Build history of the part. All positions in model axes, mm. A direction names the side the tool comes from. Round coordinates to 2 decimals unless told otherwise and drop trailing zeros. Write each loop counter-clockwise with the first axis right and the second up, starting at its lowest first coordinate (ties: lowest second). Pieces come first, ordered by that corner, then holes. Notation, with made-up numbers: (72, 76) - (78, 76) arc R30 ccw to (78, 100) - close; hole circle Ø1 at (-25.5, -23.5). An arc over 180 degrees is marked (long way). One line per question, with ' | ' between items.
Autodesk Inventor part; units mm, degrees
ref_plane "工作平面4" through (40.3, -6, 29.3998) normal (1, 0, 0) x (0, 0, -1)
ref_plane "YZ Plane" through (0, 0, 0) normal (1, 0, 0) x (0, 1, 0)
ref_plane "XZ Plane" through (0, 0, 0) normal (0, 1, 0) x (-1, 0, 0)
sketch "草圖1" plane through (0, 0, 0) normal (0, 1, 0) x (-1, 0, 0)
  line L0 (0, 0) -> (-80.6, 0)
  line L1 (-80.6, 0) -> (-80.6, 79.4)
  line L2 (-80.6, 79.4) -> (0, 79.4)
  line L3 (0, 79.4) -> (0, 0)
  line L4 (-80.6, 79.4) -> (-80.6, 51.023)
  line L5 (-80.6, 79.4) -> (-80.6, 51.023)
  line L6 (-80.6, 51.023) -> (-80.6, 79.4)
  line L7 (-94.3269, 67.1422) -> (-80.6, 79.4)
  line L8 (-96.1567, 54.4) -> (-80.6, 29.4)
  circle A0 centre (-87.6663, 59.6833) radius 3.25
  arc A1 (-94.3269, 67.1422) -> (-96.1567, 54.4) centre (-87.6663, 59.6833) ccw
  line L9 (-40.2, 92.1708) -> (-40.2, -8.9293) construction
  line L10 (0, 79.4) -> (13.727, 67.142)
  line L11 (15.5567, 54.3998) -> (0, 29.3998)
  circle A2 centre (7.0663, 59.6831) radius 3.25
  arc A3 (15.5567, 54.3998) -> (13.727, 67.142) centre (7.0663, 59.6831) ccw
  point P0 (-100.6, 61.5405)
  point P1 (20, 61.5403)
  point P2 (17.5946, 57.6964)
  point P3 (10.5946, 57.6964)
  dimension "d0" = 80.6
  dimension "d1" = 79.4
  dimension "d7" = 50
  dimension "d10" = 20
  dimension "d11" = 6.5
  dimension "d12" = 10
  dimension "d13" = 25
  dimension "d17" = 20
  dimension "d18" = 6.5
  dimension "d19" = 10
  dimension "d20" = 25
  dimension "d42" = 7
  dimension "d51" = 13.727
extrude "擠出1" add sketch "草圖1" along normal blind 2
sketch "草圖11" plane through (0, 2, 0) normal (0, 1, 0) x (1, 0, 0)
  circle A0 centre (87.6663, -59.6833) radius 3.25 construction
  line L0 (88.4163, -62.9333) -> (86.9163, -62.9333)
  line L1 (83.6663, -59.6833) -> (83.6663, -59.6833)
  line L2 (86.9163, -56.4333) -> (88.4163, -56.4333)
  line L3 (91.6663, -59.6833) -> (91.6663, -59.6833)
  arc A1 (88.4163, -62.9333) -> (91.6663, -59.6833) centre (88.4163, -59.6833) ccw
  arc A2 (91.6663, -59.6833) -> (88.4163, -56.4333) centre (88.4163, -59.6833) ccw
  arc A3 (86.9163, -56.4333) -> (83.6663, -59.6833) centre (86.9163, -59.6833) ccw
  arc A4 (83.6663, -59.6833) -> (86.9163, -62.9333) centre (86.9163, -59.6833) ccw
  point P0 (0, 0)
  dimension "d46" = 4
  dimension "d47" = 4
  dimension "d48" = 3.25
extrude "擠出5" cut sketch "草圖11" against normal through all
sketch "草圖18" plane through (0, 2, 0) normal (0, 1, 0) x (1, 0, 0)
  line L0 (0, 0) -> (-3, 0)
  line L1 (0, -29.3998) -> (-15.5567, -54.3998)
  line L2 (0, 0) -> (0, -29.3998)
  line L3 (-3, 0) -> (-3, -34.2209)
  line L4 (40.2999, -89.2199) -> (40.2999, 11.3236) construction
  line L5 (80.5999, 0) -> (83.5999, 0)
  line L6 (80.5999, 0) -> (80.5999, -29.3998)
  line L7 (83.5999, 0) -> (83.5999, -34.2209)
  line L8 (96.1567, -54.4) -> (80.6, -29.4)
  line L9 (83.5999, -34.2209) -> (80.6, -29.4)
  dimension "d60" = 3
extrude "擠出7" add sketch "草圖18" against normal blind 8 contours L2 L1 L3 L0
ref_plane "工作平面4" through (40.3, -6, 29.3998) normal (1, 0, 0) x (0, 0, -1)
mirror "鏡射2" about plane through (40.3, -6, 29.3998) normal (1, 0, 0) of "擠出7"
properties part number "mini5電腦支架"
Q1. Which spindle directions (+Z, -Z, +X, -X, +Y, -Y) get a long thin tool onto all of the face, cutting with end or side? Do faces 1 (the flat face through (88.49, 0.99, 42.08)), 2 (the flat face through (83.6, -2, 17)), 3 (the flat face through (-3, -2, 17)), 4 (the cylindrical face through (83.667, 1.014, 59.612)). Say none if no direction does.
Found:
face 1: none | face 2: -Z, +X, +Y, -Y | face 3: -Z, -X, +Y, -Y | face 4: +Y, -Y
Q2. Saw through at A-A, the plane y = -2.75. List the corners of the cut face in (x, z).
Found:
outline: (-3, 0) - (0, 0) - (0, 29.4) - (-3, 34.22) - close; (80.6, 0) - (83.6, 0) - (83.6, 34.22) - (80.6, 29.4) - close
Q3. Drill centre lines: L1, parallel to X at y = -1.75, z = 8; L2, parallel to Y at x = 51.5, z = 31; L3, parallel to X at y = 1.75, z = 15.5. Where is each one in solid material? Low to high. Write a range as from..to.
Found:
L1: -3..0, 80.6..83.6 | L2: 0..2 | L3: -3..83.6
Q4. Pull direction Z, two halves, no side cores. Call faces 5 (the flat face through (87.56, 0.986, 73.185)), 6 (the flat face through (0, -3, 14)), 7 (the flat face through (82.12, -1.94, 31.84)): +Z half, -Z half, draft (parallel to the pull), parting line (faces both ways), or undercut.
Found:
face 5: +Z half | face 6: draft | face 7: undercut
Q5. Drop flat-ended pins along their axis: pin 1 (3 mm diameter, centred on y = -3, z = 21.5, fed in from -X); pin 2 (3 mm diameter, centred on y = -1, z = 36, fed in from +X); pin 3 (4 mm diameter, centred on x = 86, y = 0, fed in from -Z). Give the stop position or say it passes through.
Found:
pin 1: x = -3 | pin 2: x = 85.4 | pin 3: z = 34.86
Q6. Saw through at C-C, the plane x = 74. List the corners of the cut face in (y, z), then the cut area to 3 significant figures.
Found:
outline: (0, 0) - (2, 0) - (2, 79.4) - (0, 79.4) - close | area: 159 mm^2
Q7. Saw through at D-D, the plane z = 73.5. List the corners of the cut face in (x, y), then the cut area to 3 significant figures.
Found:
outline: (-6.61, 0) - (87.21, 0) - (87.21, 2) - (-6.61, 2) - close | area: 188 mm^2
Q8. Saw through at B-B, the plane z = 23. List the corners of the cut face in (x, y).
Found:
outline: (-3, -6) - (0, -6) - (0, 0) - (80.6, 0) - (80.6, -6) - (83.6, -6) - (83.6, 2) - (-3, 2) - close
